The model under review builds one solid part; all positions refer to its coordinate system, in mm. Round coordinates to 2 decimals unless told otherwise and drop trailing zeros. Order: outer loops, then holes, each group sorted by start corner. A loop starts at its lowest first (then second) coordinate and runs counter-clockwise, first axis right, second up.
1) To check wall thickness, follow L1, parallel to Z at x = -16, y = -30.5; L2, parallel to Z at x = 0, y = -3.5; L3, parallel to Z at x = 0, y = -3. State the ranges of each line that lie inside material, in increasing order.
2) Consider section A-A (z = 0). Give the boundary of the cut face in (x, y), then the cut area to 3 significant figures.
3) Consider section B-B (z = 43). Give the boundary of the cut face in (x, y), then the cut area to 3 significant figures.
4) Mouldability with a two-part tool opening along Z and no side actions: class faces 1 (the face through (-25, -17, 23)), 2 (the face through (3, -4, 0)), 3 (the face through (0, -8, 0)), 4 (the face through (24, -17, 88)) as pulls with the +Z half, pulls with the -Z half, needs draft (parallel to the pull), parting line crosses it, or undercut.
from build123d import *

# Parameters (mm, degrees)
F0_W     = 50
F0_H     = 127.9575609275
F1_DEPTH = 10
F2_R     = 3
F3_DEPTH = 8
F4_DEPTH = 25
F5_SIZE  = 5
F6_SIZE  = 5
F7_SIZE  = 5
F8_SIZE  = 5
F9_R     = 5


with BuildPart() as f1:
    # F0 (on Front) → F1 (new body)
    with BuildSketch(Plane.XZ):
        with Locations((0, 26.0212195362)):
            Rectangle(F0_W, F0_H)
    extrude(amount=F1_DEPTH)

    # F2 (on face) → F3 (cut)
    with BuildSketch(Plane(origin=(0, 0, 0), x_dir=(-1, 0, 0), z_dir=(0, 1, 0))):
        Circle(F2_R)
    extrude(amount=-F3_DEPTH, mode=Mode.SUBTRACT)

    # F4 (add): a face of the model
    f4_faces = [f1.faces().sort_by_distance(p)[0] for p in [
        (0, -10, 26.0212195362),
    ]]
    extrude(f4_faces, amount=F4_DEPTH)

    # F5
    f5_edges = [f1.edges().sort_by_distance(p)[0] for p in [
        (25, 0, 26.02122),
    ]]
    chamfer(f5_edges, length=F5_SIZE)

    # F6
    f6_edges = [f1.edges().sort_by_distance(p)[0] for p in [
        (-25, 0, 26.02122),
    ]]
    chamfer(f6_edges, length=F6_SIZE)

    # F7
    f7_edges = [f1.edges().sort_by_distance(p)[0] for p in [
        (-25, -35, 26.02122),
    ]]
    chamfer(f7_edges, length=F7_SIZE)

    # F8
    f8_edges = [f1.edges().sort_by_distance(p)[0] for p in [
        (25, -35, 26.02122),
    ]]
    chamfer(f8_edges, length=F8_SIZE)

    # F9
    f9_edges = [f1.edges().sort_by_distance(p)[0] for p in [
        (0, -35, 90),
        (22.5, -32.5, 90),
        (-22.5, -32.5, 90),
        (25, -17.5, 90),
        (-25, -17.5, 90),
        (22.5, -2.5, 90),
        (-22.5, -2.5, 90),
        (0, 0, 90),
    ]]
    fillet(f9_edges, radius=F9_R)


solid = f1.part
Answer below:
1. L1: z = -37.96 to 89.97
1. L2: z = -37.96 to -3, 3 to 89.77
1. L3: z = -37.96 to -3, 3 to 89.58
2. outline: (-25, -30) - (-20, -35) - (20, -35) - (25, -30) - (25, -5) - (20, 0) - (3, 0) - (3, -8) - (-3, -8) - (-3, 0) - (-20, 0) - (-25, -5) - close
2. area: 1,650 mm2
3. outline: (-25, -30) - (-20, -35) - (20, -35) - (25, -30) - (25, -5) - (20, 0) - (-20, 0) - (-25, -5) - close
3. area: 1,700 mm2
4. face 1: needs draft
4. face 2: undercut
4. face 3: undercut
4. face 4: pulls with the +Z half
